Autodesk Fusion 360 part; units mm, degrees
sketch "Sketch1" plane through (0, 0, 0) normal (0, 1, 0) x (1, 0, 0)
  circle A0 centre (0, 0) radius 26
  circle A1 centre (0, 0) radius 32.875
  circle A2 centre (0, 0) radius 25
  circle A3 centre (0, 0) radius 33.875
  circle A4 centre (0, 0) radius 19.5
  circle A5 centre (0, 0) radius 20.5
  dimension "d1" = 67.75
  dimension "d2" = 50
  dimension "d3" = 52
  dimension "d4" = 65.75
  dimension "d10" = 39
  dimension "d25" = 41
extrude "Extrude1" add sketch "Sketch1" along normal blind 2 contours A1 | A2 | A5 makes body 1 at (30.3641, 0, 2.925) makes body 2 at (23.0736, 0, 1.242)
extrude "Extrude2" add sketch "Sketch1" along normal blind 6 bodies 2 1
sketch "Sketch2" plane through (0, 2, 0) normal (0, 1, 0) x (-1, 0, 0)
  circle A0 centre (0, 0) radius 26
  circle A1 centre (0, 0) radius 32.875
  line L0 (32, -5) -> (30.5, -5)
  line L1 (30.5, -5) -> (30.5, -1.5)
  line L2 (30.5, -1.5) -> (32, -1.5)
  line L3 (32, -1.5) -> (32, -5)
  line L4 (26.2, -1.5) -> (27.7, -1.5)
  line L5 (27.7, -1.5) -> (27.7, -5)
  line L6 (27.7, -5) -> (26.2, -5)
  line L7 (26.2, -5) -> (26.2, -1.5)
  line L8 (32, 4) -> (26, 4)
  dimension "d13" = 1.5
  dimension "d14" = 3.5
  dimension "d15" = 1.5
  dimension "d16" = 3.5
extrude "Extrude3" cut sketch "Sketch2" against normal blind 2 contours L0 L1 L2 L3 | L4 L5 L6 L7 bodies 2
ref_plane "WorkPlane1" through (-29, 2, 4) normal (0, 0.7071, 0.7071) x (1, 0, 0)
sketch "Sketch4" plane through (-29, 2, 4) normal (0, 0.7071, 0.7071) x (1, 0, 0)
  circle A0 centre (0, 0) radius 2.5
  dimension "d20" = 5
extrude "Extrude4" cut sketch "Sketch4" along normal blind 10 and the other way blind 10 bodies 2
sketch "Sketch3" plane through (0, 2, 0) normal (0, 1, 0) x (-1, 0, 0)
  line L0 (30.5, -4) -> (30.5, -0.5)
  line L1 (30.5, -0.5) -> (32, -0.5)
  line L2 (32, -0.5) -> (32, -4)
  line L3 (32, -4) -> (30.5, -4)
  line L4 (27.7, -0.5) -> (27.7, -4)
  line L5 (27.7, -4) -> (26.2, -4)
  line L6 (26.2, -4) -> (26.2, -0.5)
  line L7 (26.2, -0.5) -> (27.7, -0.5)
  circle A0 centre (0, 0) radius 26
  circle A1 centre (0, 0) radius 33
Build history of the part. All positions in model axes, mm. A direction names the side the tool comes from. Round coordinates to 2 decimals unless told otherwise and drop trailing zeros. Order: outer loops, then holes, each group sorted by start corner. A loop starts at its lowest first (then second) coordinate and runs counter-clockwise, first axis right, second up. Notation, with made-up numbers: (0.25, 42.5) -> (18.25, 42.5) arc R21 ccw to (18.25, 77.5) -> close; hole circle Ø8 at (46.5, 88). An arc over 180 degrees is marked (long way). Answer in a Markdown table with one row per item.
1) Band-saw the part on C-C on z = 15.5. Give the cut face in (x, y), and give its area (3 significant figures).
Values:
| item | result |
|---|---|
| outline | (-30.12, 0) -> (-11.83, 0) -> (-11.83, 6) -> (-13.42, 6) -> (-13.42, 2) -> (-19.62, 2) -> (-19.62, 6) -> (-20.87, 6) -> (-20.87, 2) -> (-28.99, 2) -> (-28.99, 6) -> (-30.12, 6) -> close; (11.83, 0) -> (30.12, 0) -> (30.12, 6) -> (28.99, 6) -> (28.99, 2) -> (20.87, 2) -> (20.87, 6) -> (19.62, 6) -> (19.62, 2) -> (13.42, 2) -> (13.42, 6) -> (11.83, 6) -> close |
| area | 105 mm2 |
2) Band-saw the part on D-D on z = 23.5. Give the cut face in (x, y), and give its area (3 significant figures).
Values:
| item | result |
|---|---|
| outline | (-24.4, 0) -> (24.4, 0) -> (24.4, 6) -> (22.99, 6) -> (22.99, 2) -> (11.12, 2) -> (11.12, 6) -> (8.53, 6) -> (8.53, 2) -> (-8.53, 2) -> (-8.53, 6) -> (-11.12, 6) -> (-11.12, 2) -> (-22.99, 2) -> (-22.99, 6) -> (-24.4, 6) -> close |
| area | 130 mm2 |
3) Wall check: L1, parallel to Z at x = 0, y = 4.9 (3 decimals); L2, parallel to Z at x = 4.5, y = 2.8. Give the ranges that are in metal, low to high.
Values:
| item | result |
|---|---|
| L1 | -33.875 to -32.875, -26 to -25, -20.5 to -19.5, 19.5 to 20.5, 25 to 26, 32.875 to 33.875 |
| L2 | -33.57 to -32.57, -25.61 to -24.59, -20 to -18.97, 18.97 to 20, 24.59 to 25.61, 32.57 to 33.57 |
4) Mould opens along X. For faces 4 (the flat face through (-32, 1, -3)), 5 (the flat face through (-18, 6, -28)), 6 (the cylindrical face through (-31.44, 0.63, 3.4)) say: released by +X, released by -X, zero draft, split by the parting line, or undercut.
Values:
| item | result |
|---|---|
| face 4 | undercut |
| face 5 | zero draft |
| face 6 | undercut |
5) Band-saw the part on A-A on x = 0. Give the cut face in (y, z) (3 decimals), and give its area (3 significant figures).
Values:
| item | result |
|---|---|
| outline | (0, -33.875) -> (6, -33.875) -> (6, -32.875) -> (2, -32.875) -> (2, -26) -> (6, -26) -> (6, -25) -> (2, -25) -> (2, -20.5) -> (6, -20.5) -> (6, -19.5) -> (0, -19.5) -> close; (0, 19.5) -> (6, 19.5) -> (6, 20.5) -> (2, 20.5) -> (2, 25) -> (6, 25) -> (6, 26) -> (2, 26) -> (2, 32.875) -> (6, 32.875) -> (6, 33.875) -> (0, 33.875) -> close |
| area | 81.5 mm2 |
6) Band-saw the part on B-B on y = 3.35. Give the cut face in (x, z) (3 decimals), and give its area (3 significant figures).
Values:
| item | result |
|---|---|
| outline | circle Ø67.75 at (0, 0); circle Ø52 at (0, 0); circle Ø41 at (0, 0); hole circle Ø65.75 at (0, 0); hole circle Ø50 at (0, 0); hole circle Ø39 at (0, 0) |
| area | 496 mm2 |
7) Which spindle directions (+Z, -Z, +X, -X, +Y, -Y) get a long thin tool onto all of the face, cutting with end or side? Do faces 1 (the cylindrical face through (-4.444, 3.972, -20.013)), 2 (the flat face through (15, 0, 15)), 3 (the flat face through (-31, 1, -1.5)). Say none if no direction does.
Values:
| item | result |
|---|---|
| face 1 | +Y |
| face 2 | +Z, -Z, +X, -X, -Y |
| face 3 | +Y, -Y |
8) Pin check, flat tips, straight feed: P1, Ø1, axis at y = 2, z = 23.5, coming from the -X side; P2, Ø15, axis at x = 9.5, z = 4, coming from the +Y side; P3, Ø1.2, axis at x = -31.5, y = 1, coming from the -Z side; P4, Ø0.6, axis at y = 1, z = -3.5, coming from the -X side. Stop position of each tip, or through.
Values:
| item | result |
|---|---|
| P1 | x = -24.87 |
| P2 | through |
| P3 | z = -13.88 |
| P4 | x = -33.72 |
